CAD build for the part. Positions are in the model's coordinates, mm. A direction names the side the tool comes from. Coordinates: 2 decimals unless noted, no trailing zeros. Write each loop counter-clockwise with the first axis right and the second up, starting at its lowest first coordinate (ties: lowest second). Pieces come first, ordered by that corner, then holes. Notation, with made-up numbers: (89.5, -10) -> (110.5, -10) arc R27 cw to (110.5, 19) -> close; hole circle Ø2 at (38.25, 19). An arc over 180 degrees is marked (long way). Answer as CSV lines item,"result".
```python
from build123d import *

# Parameters (mm, degrees)
SKETCH1_R           = 20.5
SKETCH1_R_2         = 17.5
BOSS_EXTRUDE1_DEPTH = 16.51
SKETCH4_R           = 17.5
SKETCH4_R_2         = 15.5


with BuildPart() as part:
    # Sketch1 → Boss-Extrude1 (new body)
    with BuildSketch(Plane.XY):
        Circle(SKETCH1_R)
        Circle(SKETCH1_R_2, mode=Mode.SUBTRACT)
    extrude(amount=BOSS_EXTRUDE1_DEPTH)

    # Sweep3: sweep along a path in Sketch5
    with BuildLine(Plane(origin=(0, 0, 0), x_dir=(1, 0, 0), z_dir=(0, 1, 0))) as sweep3_path:
        Line((0, -10.16), (0, -35.56))
        ThreePointArc((0, -35.56), (-11.159231637, -62.500768363), (-38.1, -73.66))
    # Sketch4 → Sweep3 (sweep)
    with BuildSketch(Plane.XY.offset(10.16)):
        Circle(SKETCH4_R)
        Circle(SKETCH4_R_2, mode=Mode.SUBTRACT)
    sweep(path=sweep3_path.line)


solid = part.part
```
Item 1: Two-plate mould, pull along Z, no slides. Class faces 4 (the cylindrical face through (-13.887, -10.648, 26.168)), 5 (the flat face through (-7, -14, 10.16)), 6 (the flat face through (-38.1, 12, 84)): pulls with the +Z half, pulls with the -Z half, needs draft (parallel to the pull), parting line crosses it, or undercut.
Answer below:
face 4,"undercut"
face 5,"pulls with the -Z half"
face 6,"needs draft"
Item 2: Saw through at B-B on z = 13.5. Give the cut face in (x, y), and give its area (3 significant figures).
Answer below:
outline,"circle Ø41 at (0, 0); hole circle Ø31 at (0, 0)"
area,"565 mm2"
Item 3: Flat gauge pins, fed straight in: pin 1 (21 mm diameter, centred on x = 0, y = 0, fed in from +Z); pin 2 (10 mm diameter, centred on x = -10, z = 33.5, fed in from +Y); pin 3 (1 mm diameter, centred on y = -5, z = 54.5, fed in from +X). Where does each tip first touch, or does it go through?
Answer below:
pin 1,"stops at z = 83.83"
pin 2,"stops at y = 16.77"
pin 3,"stops at x = 13.64"
Item 4: Saw through at A-A on y = 0. Give the cut face in (x, z), and give its area (3 significant figures).
Answer below:
outline,"(-38.1, 56.16) arc R20.6 cw to (-17.5, 35.56) -> (-17.5, 16.51) -> (-20.5, 16.51) -> (-20.5, 0) -> (-17.5, 0) -> (-17.5, 10.16) -> (-15.5, 10.16) -> (-15.5, 35.56) arc R22.6 ccw to (-38.1, 58.16) -> close; (-38.1, 89.16) arc R53.6 cw to (15.5, 35.56) -> (15.5, 10.16) -> (17.5, 10.16) -> (17.5, 0) -> (20.5, 0) -> (20.5, 16.51) -> (17.5, 16.51) -> (17.5, 35.56) arc R55.6 ccw to (-38.1, 91.16) -> close"
area,"440 mm2"
Item 5: Wall check: line 1 (Y direction, x = 0, z = 8); line 2 (Y direction, x = 0, z = 25.5); line 3 (Z direction, x = -7, y = -18). Give the ranges that are in metal, low to high. Write a range as from..to.
Answer below:
line 1,"y = -20.5..-17.5, 17.5..20.5"
line 2,"y = -17.5..-15.5, 15.5..17.5"
line 3,"z = 0..16.51"
Item 6: Saw through at C-C on y = -10.5. Give the cut face in (x, z), and give its area (3 significant figures).
Answer below:
outline,"(-38.1, 59.66) arc R24.1 cw to (-14, 35.56) -> (-14, 16.51) -> (-17.61, 16.51) -> (-17.61, 0) -> (-14, 0) -> (-14, 10.16) -> (-11.4, 10.16) -> (-11.4, 35.56) arc R26.7 ccw to (-38.1, 62.26) -> close; (-38.1, 85.06) arc R49.5 cw to (11.4, 35.56) -> (11.4, 10.16) -> (14, 10.16) -> (14, 0) -> (17.61, 0) -> (17.61, 16.51) -> (14, 16.51) -> (14, 35.56) arc R52.1 ccw to (-38.1, 87.66) -> close"
area,"562 mm2"
Item 7: 3-axis set-ups, long thin cutter, end or side, ignore diameter. For faces 1 (the flat face through (15.1, 9.2, 0)), 2 (the cylindrical face through (-13.887, -10.648, 5.009)), 3 (the flat face through (15.1, 9.2, 16.51)): which of +Z, -Z, +X, -X, +Y, -Y reach the whole face in a straight line?
Answer below:
face 1,"-Z, +X, -X, +Y, -Y"
face 2,"-Z"
face 3,"none"
